Here's the drawing with two shaded views (mm, measured from the low corner). I have some questions. A direction names the side the tool comes from. Give positions to 0.01 mm unless a question says otherwise; leave off trailing zeros. Write each loop counter-clockwise with the first axis right and the second up, starting at its lowest first coordinate (ties: lowest second). Pieces come first, ordered by that corner, then holes.
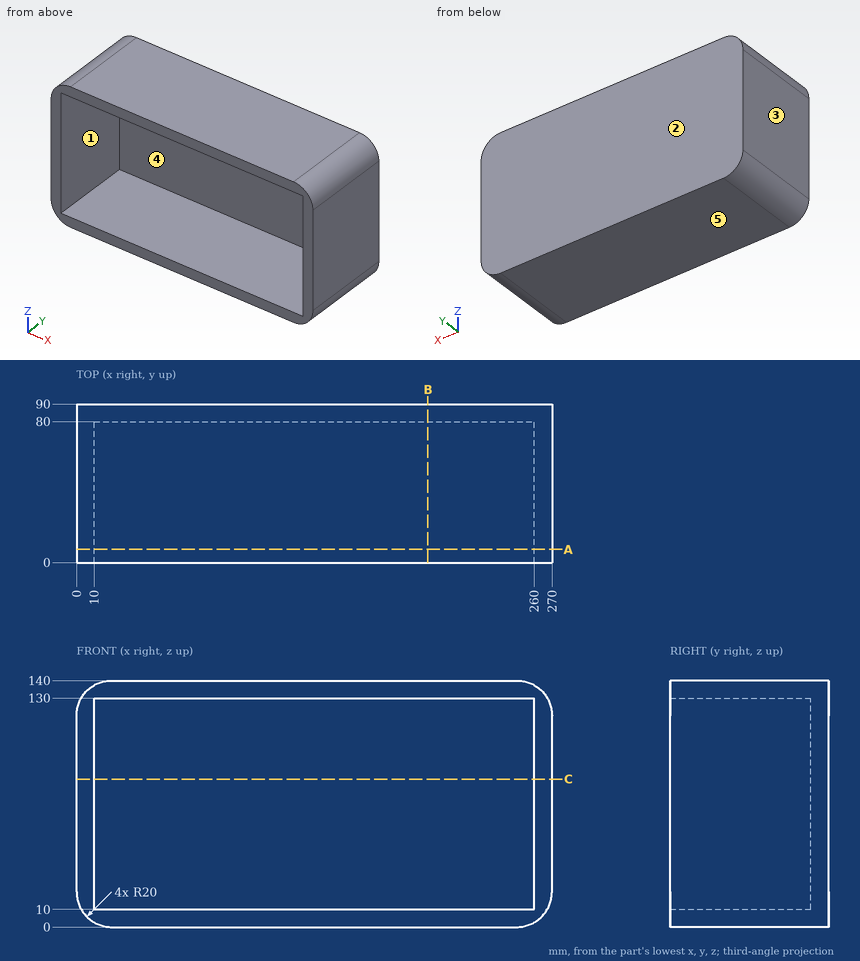
1) Suppose I cut it at A-A on y = 7.5. Write out the boundary of the cut face in (x, z), plus the area to 3 significant figures.
Values follow:
outline: (0, 20) arc R20 ccw to (20, 0) - (250, 0) arc R20 ccw to (270, 20) - (270, 120) arc R20 ccw to (250, 140) - (20, 140) arc R20 ccw to (0, 120) - close; hole (10, 10) - (260, 10) - (260, 130) - (10, 130) - close
area: 7,460 mm2
2) For pin 1 Ø4 at (x, y) = (209.5, 18) entering from -Z; pin 2 Ø12 at (x, z) = (194.5, 103.5) entering from -Y, each with a flat end and sliding along its axis, tell me the tip position at first contact or that it passes through.
Values follow:
pin 1: stops at z = 0
pin 2: stops at y = 80
3) Please list where these lines run through material, in increasing order: L1, parallel to Z at x = 217.5, y = 72; L2, parallel to X at y = 24, z = 91; L3, parallel to X at y = 74.5, z = 14.
Values follow:
L1: z = 0 to 10, 130 to 140
L2: x = 0 to 10, 260 to 270
L3: x = 0.92 to 10, 260 to 269.08
4) Suppose I cut it at B-B on x = 199.5. Write out the boundary of the cut face in (y, z), plus the area to 3 significant figures.
Values follow:
outline: (0, 0) - (90, 0) - (90, 140) - (0, 140) - (0, 130) - (80, 130) - (80, 10) - (0, 10) - close
area: 3,000 mm2
5) If we mould it in two halves opening along X, with no side actions, what happens to the marked faces 3, 4 and 5? For each: +X half, -X half, draft (parallel to the pull), parting line (faces both ways), or undercut.
Values follow:
face 3: -X half
face 4: undercut
face 5: draft
6) Suppose I cut it at C-C on z = 84. Write out the boundary of the cut face in (x, y), plus the area to 3 significant figures.
Values follow:
outline: (0, 0) - (10, 0) - (10, 80) - (260, 80) - (260, 0) - (270, 0) - (270, 90) - (0, 90) - close
area: 4,300 mm2
7) For the marked faces 1 and 2, which set-ups out of +Z, -Z, +X, -X, +Y, -Y let a thin tool reach every point of the face, with its end or its side?
Values follow:
face 1: -Y
face 2: +Z, -Z, +X, -X, +Y
